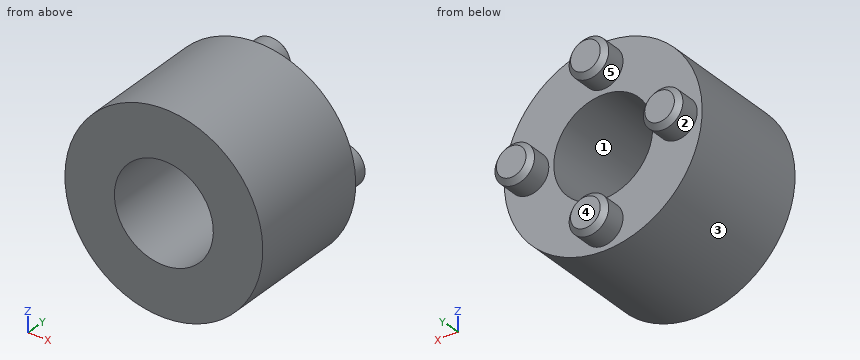
```python
from build123d import *

# Parameters (mm, degrees)
SKETCH_1_R      = 10
SKETCH_1_R_2    = 5
EXTRUDE_1_DEPTH = 13
SKETCH_2_R      = 2
EXTRUDE_2_DEPTH = 2.5
CHAMFER_1_SIZE  = 0.5


with BuildPart() as part:
    # 草图1 → 凸台-拉伸1 (new body)
    with BuildSketch(Plane(origin=(0, 0, 0), x_dir=(1, 0, 0), z_dir=(0, 1, 0))):
        with Locations(Location((0, 0, 0), (0, 0, 90))):
            Circle(SKETCH_1_R)
        with Locations(Location((0, 0, 0), (0, 0, 90))):
            Circle(SKETCH_1_R_2, mode=Mode.SUBTRACT)
    extrude(amount=EXTRUDE_1_DEPTH)

    # 草图2 → 凸台-拉伸2 (add)
    with BuildSketch(Plane(origin=(0, 13, 0), x_dir=(1, 0, 0), z_dir=(0, 1, 0))):
        with Locations(Location((0, 7.5, 0), (0, 0, 270))):
            Circle(SKETCH_2_R)
        with Locations(Location((7.5, 0, 0), (0, 0, 270))):
            Circle(SKETCH_2_R)
        with Locations(Location((0, -7.5, 0), (0, 0, 270))):
            Circle(SKETCH_2_R)
        with Locations(Location((-7.5, 0, 0), (0, 0, 270))):
            Circle(SKETCH_2_R)
    extrude(amount=EXTRUDE_2_DEPTH)

    # 倒角1
    chamfer_1_edges = [part.edges().sort_by_distance(p)[0] for p in [
        (0, 15.5, -9.5),
        (7.5, 15.5, -2),
        (0, 15.5, 5.5),
        (-7.5, 15.5, -2),
    ]]
    chamfer(chamfer_1_edges, length=CHAMFER_1_SIZE)


solid = part.part
```
Geometry: final body of the model. Coordinates: model frame, mm. Face numbers are marked on the shaded views. A direction names the side the tool comes from. Coordinates: 2 decimals unless noted, no trailing zeros. Write each loop counter-clockwise with the first axis right and the second up, starting at its lowest first coordinate (ties: lowest second). Pieces come first, ordered by that corner, then holes. Notation, with made-up numbers: M 48,-11.75 L 57,-11.75 A14 cw 57,-3.75 Z; hole C -30,-23 d3. An arc over 180 degrees is marked long. Answer as CSV lines item,"result". Start each with the question number.
Q1. Reachability of the marked faces 1 and 2 from +Z, -Z, +X, -X, +Y, -Y: full face, straight path, thin tool, end or side. Return the list, or none.
Q2. Cut plane C-C on y = 6.5. Return the cut outline in (x, z), then the cut area to 3 significant figures.
Q3. Line query: line 1 (X direction, y = 5, z = 0); line 2 (Y direction, x = -5, z = 7.25); line 3 (X direction, y = 1.75, z = -3.5). Output: solid intervals per line, ascending. Write a range as from..to.
Q4. Cut plane B-B on z = 0. Return the cut outline in (x, y).
Q5. Mould query, pull axis Z, two halves, no side actions, for the marked faces 3, 4 and 5. Classes: released by +Z, released by -Z, zero draft, split by the parting line, or undercut.
Q6. Cut plane A-A on x = 0. Return the cut outline in (y, z).
Q7. Pin query (flat end, axial travel): P1, Ø4, axis at x = 2.5, z = 0.5, coming from the -Y side; P2, Ø1, axis at y = 9.5, z = -6.5, coming from the +X side; P3, Ø2, axis at x = 5, y = 6, coming from the +Z side; P4, Ø2, axis at x = -7.5, y = 7.5, coming from the +Z side. Return the tip coordinate at first contact, or that it passes through.
Q8. Cut plane D-D on y = 13.5. Return the cut outline in (x, z), then the cut area to 3 significant figures.
Findings below:
1,face 1,"+Y, -Y"
1,face 2,"+Y"
2,outline,"C 0,0 d20; hole C 0,0 d10"
2,area,"236 mm2"
3,line 1,"x = -10..-5, 5..10"
3,line 2,"y = 0..13"
3,line 3,"x = -9.37..-3.57, 3.57..9.37"
4,outline,"M -10,0 L -5,0 L -5,13 L -5.5,13 L -5.5,15 L -6,15.5 L -9,15.5 L -9.5,15 L -9.5,13 L -10,13 Z; M 5,0 L 10,0 L 10,13 L 9.5,13 L 9.5,15 L 9,15.5 L 6,15.5 L 5.5,15 L 5.5,13 L 5,13 Z"
5,face 3,"split by the parting line"
5,face 4,"zero draft"
5,face 5,"undercut"
6,outline,"M 0,-10 L 13,-10 L 13,-9.5 L 15,-9.5 L 15.5,-9 L 15.5,-6 L 15,-5.5 L 13,-5.5 L 13,-5 L 0,-5 Z; M 0,5 L 13,5 L 13,5.5 L 15,5.5 L 15.5,6 L 15.5,9 L 15,9.5 L 13,9.5 L 13,10 L 0,10 Z"
7,P1,"passes through"
7,P2,"stops at x = 8"
7,P3,"stops at z = 9.17"
7,P4,"stops at z = 7.6"
8,outline,"C -7.5,0 d4; C 0,-7.5 d4; C 0,7.5 d4; C 7.5,0 d4"
8,area,"50.3 mm2"
